The model under review builds one solid part; all positions refer to its coordinate system, in mm. A direction names the side the tool comes from. Give positions to 0.01 mm unless a question says otherwise; leave off trailing zeros. Write each loop counter-clockwise with the first axis right and the second up, starting at its lowest first coordinate (ties: lowest second). Pieces come first, ordered by that corner, then holes.
from build123d import *

# Parameters (mm, degrees)
BOSS_EXTRUDE1_DEPTH = 52.5
CUT_EXTRUDE1_START  = -20
SKETCH2_R           = 37.5
CUT_EXTRUDE1_DEPTH  = 20
BOSS_EXTRUDE2_DEPTH = 12.5
BOSS_EXTRUDE3_DEPTH = 12.5


with BuildPart() as part:
    # Sketch1 → Boss-Extrude1 (new body, symmetric)
    with BuildSketch(Plane.XY):
        with BuildLine():
            Line((45, 0), (105, 0))
            Line((105, 0), (105, 60))
            Line((105, 60), (80, 60))
            Line((80, 60), (80, 140))
            Line((80, 140), (20, 140))
            Line((20, 140), (20, 120))
            Line((20, 120), (45, 120))
            Line((45, 120), (45, 90))
            Line((45, 90), (-45, 90))
            Line((-45, 90), (-45, 120))
            Line((-45, 120), (-20, 120))
            Line((-20, 120), (-20, 140))
            Line((-20, 140), (-80, 140))
            Line((-80, 140), (-80, 60))
            Line((-80, 60), (-105, 60))
            Line((-105, 60), (-105, 0))
            Line((-105, 0), (-45, 0))
            ThreePointArc((-45, 0), (0, 45), (45, 0))
        make_face()
    extrude(amount=BOSS_EXTRUDE1_DEPTH, both=True)

    # Sketch2 → Cut-Extrude1 (cut)
    with BuildSketch(Plane(origin=(0, 140, 0), x_dir=(1, 0, 0), z_dir=(0, 1, 0)).offset(CUT_EXTRUDE1_START)):
        Circle(SKETCH2_R)
    extrude(amount=CUT_EXTRUDE1_DEPTH, mode=Mode.SUBTRACT)

    # Sketch3 → Boss-Extrude2 (add, symmetric)
    with BuildSketch(Plane.XY):
        Polygon((105, 60), (80, 60), (80, 140), align=None)
    extrude(amount=BOSS_EXTRUDE2_DEPTH, both=True)

    # Sketch4 → Boss-Extrude3 (add, symmetric)
    with BuildSketch(Plane.XY):
        Polygon((-105, 60), (-80, 60), (-80, 140), align=None)
    extrude(amount=BOSS_EXTRUDE3_DEPTH, both=True)


solid = part.part
1) The part is to be moulded in two halves that separate along Y. For faces 4 (the flat face through (-50, 140, 1)), 5 (the flat face through (38, 120, 1)), 6 (the flat face through (20, 130, -42)), say which applies: +Y half, -Y half, draft (parallel to the pull), parting line (faces both ways), or undercut.
2) Tool access review of faces 1 (the flat face through (-38, 120, 1)), 2 (the flat face through (-20, 130, -42)), 3 (the flat face through (87, 83, -12.5)): name each direction out of +Z, -Z, +X, -X, +Y, -Y from which nothing blocks a thin tool from reaching the whole face with its end or side.
3) To check wall thickness, follow probe 1 along X at (y, z) = (100, -43); probe 2 along Z at (x, y) = (83.5, 78); probe 3 along Y at (x, z) = (21, 35). State the ranges of each line that lie inside material, in increasing order.
4) Insertion check: pin 1 (7.5 mm diameter, centred on x = -93.5, z = 39.5, fed in from +Y); pin 2 (12.5 mm diameter, centred on x = -88.5, y = 94.5, fed in from +Z); pin 3 (10 mm diameter, centred on y = 134, z = 46.5, fed in from +X). Each pin has a flat end and moves straight along its axis. Give the tip position at first contact, or say it passes through.
5) Consider section C-C, the plane z = -34. Give the boundary of the cut face in (x, y), then the cut area to 3 significant figures.
6) Consider section B-B, the plane x = -31. Give the boundary of the cut face in (y, z).
7) Consider section A-A, the plane y = 107.5. Give the boundary of the cut face in (x, z).
8) Consider section D-D, the plane y = 40. Give the boundary of the cut face in (x, z), then the cut area to 3 significant figures.
Answer block:
1. face 4: +Y half
1. face 5: undercut
1. face 6: draft
2. face 1: +Z, -Z
2. face 2: +Z, -Z, +Y
2. face 3: -Z, +X, +Y
3. probe 1: x = -80 to -45, 45 to 80
3. probe 2: z = -12.5 to 12.5
3. probe 3: y = 39.8 to 90, 120 to 140
4. pin 1: stops at y = 60
4. pin 2: stops at z = 12.5
4. pin 3: stops at x = 80
5. outline: (-105, 0) - (-45, 0) arc R45 cw to (45, 0) - (105, 0) - (105, 60) - (80, 60) - (80, 140) - (20, 140) - (20, 120) - (45, 120) - (45, 90) - (-45, 90) - (-45, 120) - (-20, 120) - (-20, 140) - (-80, 140) - (-80, 60) - (-105, 60) - close
5. area: 18,700 mm2
6. outline: (32.62, -52.5) - (90, -52.5) - (90, 52.5) - (32.62, 52.5) - close; (120, -52.5) - (140, -52.5) - (140, -21.1) - (120, -21.1) - close; (120, 21.1) - (140, 21.1) - (140, 52.5) - (120, 52.5) - close
7. outline: (-90.16, -12.5) - (-80, -12.5) - (-80, -52.5) - (-45, -52.5) - (-45, 52.5) - (-80, 52.5) - (-80, 12.5) - (-90.16, 12.5) - close; (45, -52.5) - (80, -52.5) - (80, -12.5) - (90.16, -12.5) - (90.16, 12.5) - (80, 12.5) - (80, 52.5) - (45, 52.5) - close
8. outline: (-105, -52.5) - (-20.62, -52.5) - (-20.62, 52.5) - (-105, 52.5) - close; (20.62, -52.5) - (105, -52.5) - (105, 52.5) - (20.62, 52.5) - close
8. area: 17,700 mm2
